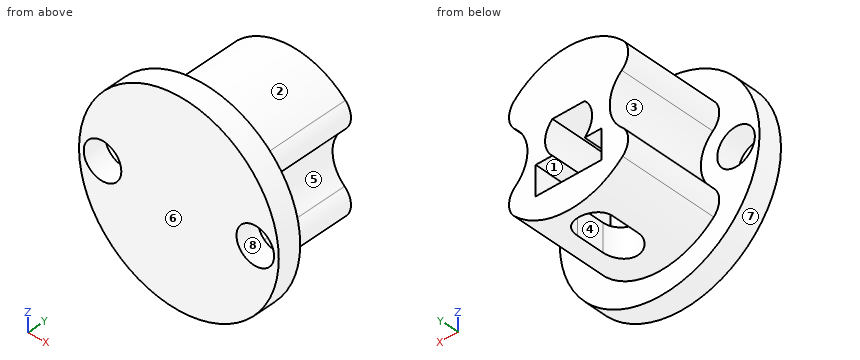
Autodesk Inventor part; units mm, degrees
ref_plane "Work Plane1" through (-2.8, 7, -8.95) normal (0, 0, 1) x (1, 0, 0)
ref_plane "YZ Plane" through (0, 0, 0) normal (1, 0, 0) x (0, 1, 0)
ref_plane "XZ Plane" through (0, 0, 0) normal (0, 1, 0) x (-1, 0, 0)
sketch "Sketch1" plane through (0, 0, 0) normal (0, 1, 0) x (-1, 0, 0)
  circle A0 centre (0, 0) radius 4.5
  circle A1 centre (0, 0) radius 2
  circle A2 centre (0, 0) radius 1.45
  line L0 (0, -1.45) -> (1.3775, -1.45)
  line L1 (0, -1.45) -> (-1.3775, -1.45)
  line L2 (0, 1.45) -> (-1.3775, 1.45)
  line L3 (0, 1.45) -> (1.3775, 1.45)
  dimension "d0" = 9
  dimension "d1" = 4
  dimension "d2" = 2.9
extrude "Extrusion1" add sketch "Sketch1" along normal blind 7 contours A0 | L3 L2 A1 | A1 L1 L0
sketch "Sketch2" plane through (0, 7, 0) normal (0, 1, 0) x (1, 0, 0)
  line L0 (-1.3775, 1.45) -> (1.3775, 1.45)
  line L1 (0, 1.45) -> (0, 3.85)
  line L2 (1.3775, -0.95) -> (-1.3775, -0.95)
  line L3 (-1.3775, -0.95) -> (-1.3775, 3.85)
  line L4 (-1.3775, 3.85) -> (1.3775, 3.85)
  line L5 (1.3775, 3.85) -> (1.3775, -0.95)
  line L6 (1.3775, -0.95) -> (-1.3775, 3.85) construction
  line L7 (-1.3775, -0.95) -> (1.3775, 3.85) construction
  line L8 (2.75, -0.95) -> (-2.75, -0.95)
  line L9 (-2.75, -0.95) -> (-2.75, 3.85)
  line L10 (-2.75, 3.85) -> (2.75, 3.85)
  line L11 (2.75, 3.85) -> (2.75, -0.95)
  line L12 (2.75, -0.95) -> (-2.75, 3.85) construction
  line L13 (-2.75, -0.95) -> (2.75, 3.85) construction
  circle A0 centre (0, 0) radius 6.5
  circle A1 centre (0, 0) radius 4.5
  dimension "d5" = 2.4
  dimension "d6" = 5.5
  dimension "d7" = 13
extrude "Extrusion2" add sketch "Sketch2" against normal blind 7 contours A1 L9 L10 | L10 L11 A1 | A0
sketch "Sketch3" plane through (0, 7, 0) normal (0, 1, 0) x (1, 0, 0)
  line L0 (-1.3775, 1.45) -> (1.3775, 1.45)
  line L1 (0, 1.45) -> (0, 3.95)
  line L2 (2.8, -1.05) -> (-2.8, -1.05)
  line L3 (-2.8, -1.05) -> (-2.8, 3.95)
  line L4 (-2.8, 3.95) -> (2.8, 3.95)
  line L5 (2.8, 3.95) -> (2.8, -1.05)
  line L6 (2.8, -1.05) -> (-2.8, 3.95) construction
  line L7 (-2.8, -1.05) -> (2.8, 3.95) construction
  line L8 (0, 1.45) -> (-2.8, 1.45)
  line L9 (0, 1.45) -> (2.8, 1.45)
  point P0 (0, 0)
  dimension "d10" = 2.5
  dimension "d11" = 5.6
extrude "Extrusion3" cut sketch "Sketch3" against normal blind 7 contours L8 L3 L4 L1 L0 | L1 L4 L5 L9 L0
ref_plane "Work Plane1" through (-2.8, 7, -8.95) normal (0, 0, 1) x (1, 0, 0)
sketch "Sketch5" plane through (-2.8, 7, -8.95) normal (0, 0, 1) x (1, 0, 0)
  circle A0 centre (2.8, -2.4541) radius 1.5
  line L0 (2.8, -2.4541) -> (2.8, -7)
  circle A1 centre (2.8, -3.9541) radius 1.5
  circle A2 centre (2.8, -4.8651) radius 1.5
  line L1 (1.3, -4.8651) -> (1.3, -2.4541)
  line L2 (4.3, -4.8651) -> (4.3, -2.4541)
  point P0 (4.3, -4.8651)
  dimension "d17" = 3
  dimension "d15" = 3
  dimension "d16" = 3
extrude "Extrusion4" cut sketch "Sketch5" along normal blind 6
sketch "Sketch6" plane through (0, 0, 0) normal (0, -1, 0) x (1, 0, 0)
  circle A0 centre (0, 0) radius 6.5
extrude "Extrusion5" add sketch "Sketch6" along normal blind 1.5
sketch "Sketch7" plane through (0, -1.5, 0) normal (0, -1, 0) x (1, 0, 0)
  line L0 (-3.5, -3.5) -> (3.5, -3.5)
  line L1 (3.5, -3.5) -> (3.5, 3.5)
  line L2 (3.5, 3.5) -> (-3.5, 3.5)
  line L3 (-3.5, 3.5) -> (-3.5, -3.5)
  line L4 (-3.5, -3.5) -> (3.5, 3.5) construction
  line L5 (3.5, -3.5) -> (-3.5, 3.5) construction
  point P0 (0, 0)
  dimension "d22" = 7
  dimension "d23" = 7
extrude "Extrusion6" add sketch "Sketch7" along normal blind 6
sketch "Sketch8" plane through (0, -1.5, 0) normal (0, -1, 0) x (1, 0, 0)
  arc A0 (-1.3775, 1.45) -> (-1.3775, -1.45) centre (0, 0) ccw
  circle A1 centre (0, 0) radius 8.6758
extrude "Extrusion7" cut sketch "Sketch8" along normal blind 10
sketch "Sketch9" plane through (0, -1.5, 0) normal (0, -1, 0) x (1, 0, 0)
  point P0 (0, 0)
sketch "Sketch10" plane through (0, -1.5, 0) normal (0, -1, 0) x (1, 0, 0)
  circle A0 centre (0, 0) radius 6.5
  circle A1 centre (6.5, 0) radius 3
  circle A2 centre (-6.5, 0) radius 3
  dimension "d28" = 13
  dimension "d29" = 6
  dimension "d30" = 6
extrude "Extrusion8" cut sketch "Sketch10" against normal through all contours A0 A1 | A0 A1 | A2 A0 | A0 A2
sketch "Sketch11" plane through (0, -1.5, 0) normal (0, -1, 0) x (1, 0, 0)
  circle A0 centre (0, 0) radius 8.5
  dimension "d33" = 17
extrude "Extrusion9" add sketch "Sketch11" along normal blind 2
sketch "Sketch12" plane through (0, -3.5, 0) normal (0, -1, 0) x (1, 0, 0)
  arc A0 (1.3775, -1.45) -> (1.3775, 1.45) centre (0, 0) ccw
  circle A1 centre (0, 0) radius 6.5
  arc A2 (-5.8077, -2.919) -> (-5.8077, 2.919) centre (-6.5, 0) ccw
  circle A3 centre (-6.5, 0) radius 1.6
  circle A4 centre (6.5, 0) radius 1.6
  dimension "d36" = 13
  dimension "d37" = 3.2
  dimension "d38" = 3.2
extrude "Extrusion10" cut sketch "Sketch12" against normal through all contours A1 A4 | A1 A4 | A3 A1 | A1 A3
fillet "Fillet1" radius 1.6 4 edges at (5.8077, 2.75, 2.919) (5.8077, 2.75, -2.919) (-5.8077, 2.75, 2.919) (-5.8077, 2.75, -2.919)
properties part number "acople"
For this review, take the finished solid that the model builds, in its own axes (mm). Face numbers are marked on the shaded views. A direction names the side the tool comes from. Round coordinates to 2 decimals unless told otherwise and drop trailing zeros. Order: outer loops, then holes, each group sorted by start corner. A loop starts at its lowest first (then second) coordinate and runs counter-clockwise, first axis right, second up.
Q1. Mouldability with a two-part tool opening along X and no side actions: class the marked faces 5, 6, 7 and 8 as pulls with the +X half, pulls with the -X half, needs draft (parallel to the pull), parting line crosses it, or undercut.
Findings below:
face 5: pulls with the +X half
face 6: needs draft
face 7: parting line crosses it
face 8: undercut
Q2. We need section B-B, the plane z = 0. Give the boundary of the cut face in (x, y).
Findings below:
outline: (-8.5, -3.5) - (-8.1, -3.5) - (-8.1, -1.5) - (-8.5, -1.5) - close; (-4.9, -3.5) - (4.9, -3.5) - (4.9, -1.5) - (3.5, -1.5) - (3.5, 7) - (2, 7) - (2, 0) - (-2, 0) - (-2, 7) - (-3.5, 7) - (-3.5, -1.5) - (-4.9, -1.5) - close; (8.1, -3.5) - (8.5, -3.5) - (8.5, -1.5) - (8.1, -1.5) - close
Q3. We need section A-A, the plane x = 0. Give the boundary of the cut face in (y, z), plus the area to 3 significant figures.
Findings below:
outline: (-3.5, -8.5) - (-1.5, -8.5) - (-1.5, -6.5) - (0.63, -6.5) - (0.63, -3.95) - (0, -3.95) - (0, 1.45) - (7, 1.45) - (7, 6.5) - (-1.5, 6.5) - (-1.5, 8.5) - (-3.5, 8.5) - close; (6.05, -6.5) - (7, -6.5) - (7, -3.95) - (6.05, -3.95) - close
area: 92.9 mm2
Q4. Insertion check: P1, Ø1.9, axis at y = 3, z = -5.5, coming from the -X side; P2, Ø3.5, axis at x = 6.5, z = 0, coming from the +Y side; P3, Ø1, axis at y = 2.5, z = -3.5, coming from the +X side. Each pin has a flat end and moves straight along its axis. Give the tip position at first contact, or say it passes through.
Findings below:
P1: stops at x = -4.64
P2: stops at y = -1.5
P3: stops at x = 5.07
Q5. Machinability: for the marked faces 1, 2, 3 and 4, which of the approach directions +Z, -Z, +X, -X, +Y, -Y give a long, thin tool a straight path to every point of the face, cutting with its end or side? Answer none if there is none.
Findings below:
face 1: +Y
face 2: +Z, +Y
face 3: -X, +Y
face 4: -Z
Q6. We need section C-C, the plane z = -5.25. Give the boundary of the cut face in (x, y), plus the area to 3 significant figures.
Findings below:
outline: (-6.68, -3.5) - (6.68, -3.5) - (6.68, -1.5) - (3.83, -1.5) - (3.83, 7) - (-3.83, 7) - (-3.83, -1.5) - (-6.68, -1.5) - close; hole (-1.5, 2.13) arc R1.5 ccw to (1.5, 2.13) - (1.5, 4.55) arc R1.5 ccw to (-1.5, 4.55) - close
area: 77.6 mm2
Q7. We need section D-D, the plane x = -6.5. Give the boundary of the cut face in (y, z), plus the area to 3 significant figures.
Findings below:
outline: (-3.5, -5.48) - (-1.5, -5.48) - (-1.5, -1.6) - (-3.5, -1.6) - close; (-3.5, 1.6) - (-1.5, 1.6) - (-1.5, 5.48) - (-3.5, 5.48) - close
area: 15.5 mm2
Q8. Wall thickness on line 1 (Y direction, x = 5.5, z = 5); line 2 (Z direction, x = -2.25, y = 1.75); line 3 (Z direction, x = 6.5, y = -2.6): over which ranges is each line inside the solid? List them lowest first.
Findings below:
line 1: y = -3.5 to -1.5
line 2: z = -6.1 to -3.95, -1.45 to 6.1
line 3: z = -5.48 to -1.6, 1.6 to 5.48
